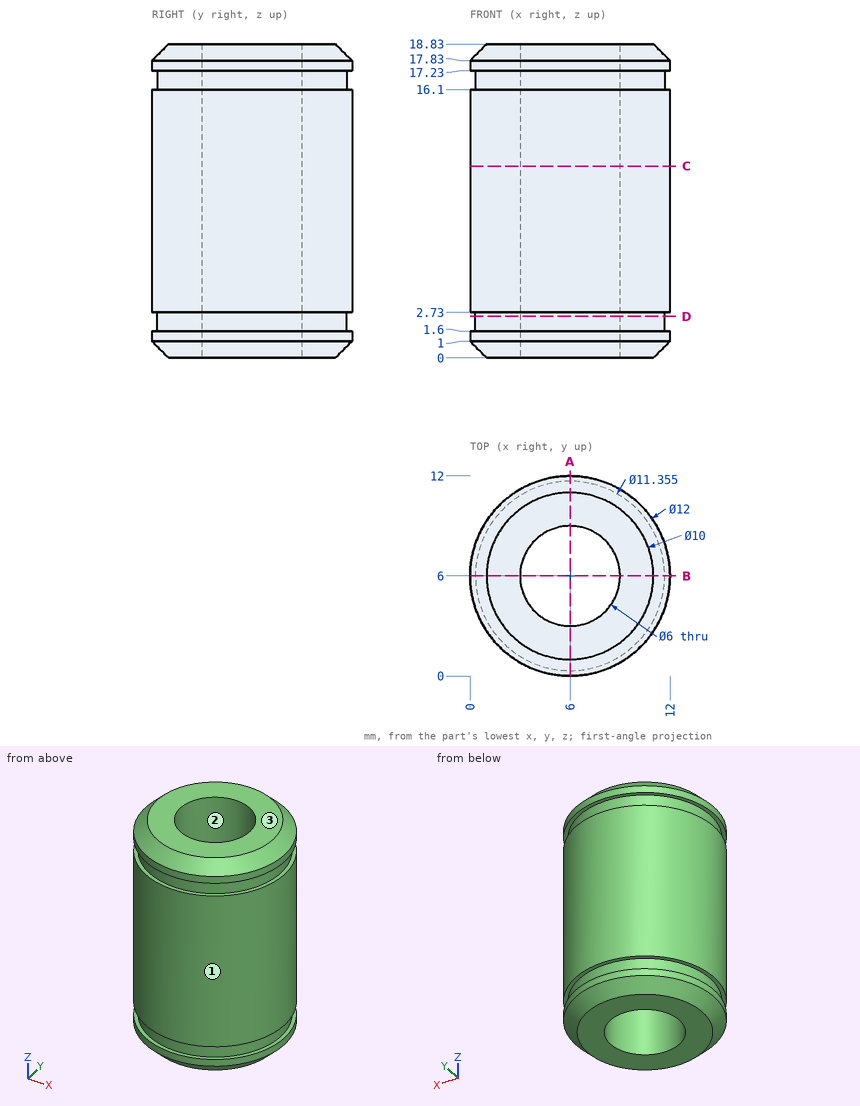
Could you check a few things on this drawing? It's one solid part, dimensions in mm from its lowest x, y, z. Give positions to 0.01 mm unless a question says otherwise; leave off trailing zeros. Write each loop counter-clockwise with the first axis right and the second up, starting at its lowest first coordinate (ties: lowest second). Pieces come first, ordered by that corner, then holes. Notation, with made-up numbers: (10.5, 24) -> (25.5, 24) arc R16 cw to (25.5, 39) -> close; hole circle Ø5 at (-2.75, 6). An arc over 180 degrees is marked (long way). Answer as CSV lines item,"result". Start each with the question number.
(1) If we mould it in two halves opening along Y, with no side actions, what happens to the marked faces 1, 2 and 3? For each: +Y half, -Y half, draft (parallel to the pull), parting line (faces both ways), or undercut.
(2) If we section it at C-C, the plane z = 11.5: Write out the boundary of the cut face in (x, y).
(3) Please list where these lines run through material, in increasing order: line 1 (Y direction, x = 6, z = 8.75); line 2 (X direction, y = 4, z = 12) (1 decimal); line 3 (Y direction, x = 4.5, z = 11.25).
(4) If we section it at D-D, the plane z = 2.5: Write out the boundary of the cut face in (x, y) (1 decimal).
(5) I'm going to push a flat-ended pin straight in: pin 1 Ø5 at (x, z) = (1.5, 16) entering from +Y. Where does the tip first touch, or does it pass through?
(6) If we section it at A-A, the plane x = 6: Write out the boundary of the cut face in (y, z).
Answer list:
1,face 1,"parting line"
1,face 2,"undercut"
1,face 3,"draft"
2,outline,"circle Ø12 at (6, 6); hole circle Ø6 at (6, 6)"
3,line 1,"0 to 3, 9 to 12"
3,line 2,"0.3 to 3.8, 8.2 to 11.7"
3,line 3,"0.19 to 3.4, 8.6 to 11.81"
4,outline,"circle Ø11.4 at (6, 6); hole circle Ø6 at (6, 6)"
5,pin 1,"y = 11.66"
6,outline,"(0, 1) -> (1, 0) -> (3, 0) -> (3, 18.83) -> (1, 18.83) -> (0, 17.83) -> (0, 17.23) -> (0.32, 17.23) -> (0.32, 16.1) -> (0, 16.1) -> (0, 2.73) -> (0.32, 2.73) -> (0.32, 1.6) -> (0, 1.6) -> close; (9, 0) -> (11, 0) -> (12, 1) -> (12, 1.6) -> (11.68, 1.6) -> (11.68, 2.73) -> (12, 2.73) -> (12, 16.1) -> (11.68, 16.1) -> (11.68, 17.23) -> (12, 17.23) -> (12, 17.83) -> (11, 18.83) -> (9, 18.83) -> close"
